The model under review builds one solid part; all positions refer to its coordinate system, in mm. Round coordinates to 2 decimals unless told otherwise and drop trailing zeros. Loops run counter-clockwise (first coordinate to the right, second up) from the corner with the lowest first, then second, coordinate; pieces in that order, holes last. Notation, with made-up numbers: (-24.75, 33) -> (16.25, 33) arc R10 cw to (16.25, 47) -> close; hole circle Ø9 at (87, 67). An arc over 180 degrees is marked (long way). Use a Markdown table: item, result. Add a question column.
1) Consider section C-C on x = 0.3. Give the boundary of the cut face in (y, z).
2) Consider section D-D on z = -4.6. Give the boundary of the cut face in (x, y), plus the area to 3 significant figures.
3) Mouldability with a two-part tool opening along Y and no side actions: class faces 1 (the flat face through (0.25, 18.53, -4.26)), 2 (the flat face through (0.5, 10.4, -2.5)), 3 (the cylindrical face through (0.25, 10.18, -2.34)) as released by +Y, released by -Y, zero draft, split by the parting line, or undercut.
4) Wall thickness on probe 1 along Y at (x, z) = (0.1, -2.5); probe 2 along Z at (x, y) = (0.45, 8.5); probe 3 along Z at (x, y) = (0.45, 10): over which ranges is each line inside the solid? List them lowest first.
5) Consider section A-A on z = -2.5. Give the boundary of the cut face in (x, y), plus the area to 3 significant figures.
6) Consider section B-B on y = 3. Give the boundary of the cut face in (x, z).
from build123d import *

# Parameters (mm, degrees)
SKETCH_1_W             = 5
SKETCH_1_H             = 20.5
EXTRUDE_1_DEPTH        = 0.5
HOLE_WIZARD_21_D       = 2.38252
CHAMFER_1_SIZE         = 4
CHAMFER_1_SIZE2        = 1.455880937
CHAMFER_1_PART_2_SIZE  = 4
CHAMFER_1_PART_2_SIZE2 = 1.455880937


with BuildPart() as part:
    # Эскиз1 → Бобышка-Вытянуть1 (new body)
    with BuildSketch(Plane(origin=(0, 0, 0), x_dir=(0, 0, -1), z_dir=(1, 0, 0))):
        with Locations((2.5, 10.25)):
            Rectangle(SKETCH_1_W, SKETCH_1_H)
    extrude(amount=EXTRUDE_1_DEPTH)

    # Сверло под метчик  спиральное #21 (through all)
    with Locations(Plane.ZY):
        with Locations((-2.5, 3), (-2.5, 9)):
            Hole(HOLE_WIZARD_21_D / 2)

    # Фаска1
    chamfer_1_edges = [part.edges().sort_by_distance(p)[0] for p in [
        (0.25, 20.5, 0),
    ]]
    chamfer_1_side = [part.faces().sort_by_distance(p)[0] for p in [
        (0.25, 10.25, 0),
    ]]
    chamfer(chamfer_1_edges, length=CHAMFER_1_SIZE, length2=CHAMFER_1_SIZE2, reference=chamfer_1_side[0])

    # Фаска1 part 2
    chamfer_1_part_2_edges = [part.edges().sort_by_distance(p)[0] for p in [
        (0.25, 20.5, -5),
    ]]
    chamfer_1_part_2_side = [part.faces().sort_by_distance(p)[0] for p in [
        (0.25, 10.25, -5),
    ]]
    chamfer(chamfer_1_part_2_edges, length=CHAMFER_1_PART_2_SIZE, length2=CHAMFER_1_PART_2_SIZE2, reference=chamfer_1_part_2_side[0])


solid = part.part
Result set:
| question | item | result |
|---|---|---|
| 1 | outline | (0, -5) -> (16.5, -5) -> (20.5, -3.54) -> (20.5, -1.46) -> (16.5, 0) -> (0, 0) -> close; hole circle Ø2.38 at (3, -2.5); hole circle Ø2.38 at (9, -2.5) |
| 2 | outline | (0, 0) -> (0.5, 0) -> (0.5, 17.6) -> (0, 17.6) -> close |
| 2 | area | 8.80 mm2 |
| 3 | face 1 | released by +Y |
| 3 | face 2 | zero draft |
| 3 | face 3 | undercut |
| 4 | probe 1 | 0 to 1.81, 4.19 to 7.81, 10.19 to 20.5 |
| 4 | probe 2 | -5 to -3.58, -1.42 to 0 |
| 4 | probe 3 | -5 to -3.15, -1.85 to 0 |
| 5 | outline | (0, 0) -> (0.5, 0) -> (0.5, 1.81) -> (0, 1.81) -> close; (0, 4.19) -> (0.5, 4.19) -> (0.5, 7.81) -> (0, 7.81) -> close; (0, 10.19) -> (0.5, 10.19) -> (0.5, 20.5) -> (0, 20.5) -> close |
| 5 | area | 7.87 mm2 |
| 6 | outline | (0, -5) -> (0.5, -5) -> (0.5, -3.69) -> (0, -3.69) -> close; (0, -1.31) -> (0.5, -1.31) -> (0.5, 0) -> (0, 0) -> close |
